Could you check a few things on this model? Use its own coordinates, in mm. A direction names the side the tool comes from. Give positions to 0.01 mm unless a question says otherwise; leave off trailing zeros. Loops run counter-clockwise (first coordinate to the right, second up) from the corner with the lowest first, then second, coordinate; pieces in that order, holes last. Notation, with made-up numbers: M -31.5,61 L 14.5,61 A31 ccw 14.5,86 Z; hole C 50,36 d7. An arc over 180 degrees is marked long. Answer in a Markdown table with one row per item. Add a question column.
```python
from build123d import *

# Parameters (mm, degrees)
F0_W          = 38
F0_H          = 18.5
F0_R          = 1.5
F0_W_2        = 10
F0_R_2        = 1.75
F1_DEPTH      = 5
F2_W          = 25
F2_H          = 18.5
F3_DEPTH      = 5
F5_DEPTH      = 41.501
F5_DEPTH_BACK = 16.501


with BuildPart() as f1:
    # F0 (on Top) → F1 (new body)
    with BuildSketch(Plane.XY):
        Rectangle(F0_W, F0_H)
        with Locations((-16.65, 0)):
            Circle(F0_R, mode=Mode.SUBTRACT)
        with Locations((16.65, 0)):
            Circle(F0_R, mode=Mode.SUBTRACT)
        with Locations((24, 0)):
            Rectangle(F0_W_2, F0_H)
        with Locations((25, 0)):
            Circle(F0_R_2, mode=Mode.SUBTRACT)
        with Locations((-24, 0)):
            Rectangle(F0_W_2, F0_H)
        with Locations((-25, 0)):
            Circle(F0_R_2, mode=Mode.SUBTRACT)
    extrude(amount=F1_DEPTH)

    # F2 (on face) → F3 (join)
    with BuildSketch(Plane.XY.offset(5)):
        Rectangle(F2_W, F2_H)
    extrude(amount=F3_DEPTH)

    # F4 (on face) → F5 (cut, two sides)
    with BuildSketch(Plane(origin=(-12.5, 0, 0), x_dir=(0, -1, 0), z_dir=(-1, 0, 0))) as f5_sk:
        Polygon((-4.625, 5), (0, 10), (-9.25, 10), (-9.25, 5), align=None)
        Polygon((9.25, 10), (0, 10), (4.625, 5), (9.25, 5), align=None)
        Polygon((9.25, 5), (4.625, 5), (9.25, 0), align=None)
        Polygon((-9.25, 0), (-4.625, 5), (-9.25, 5), align=None)
    extrude(amount=-F5_DEPTH, mode=Mode.SUBTRACT)
    extrude(f5_sk.sketch, amount=F5_DEPTH_BACK, mode=Mode.SUBTRACT)


solid = f1.part
```
Item 1: For faces 4 (the face through (-18.15, 0.07, 2.46)), 5 (the face through (-12.5, 0, 7)), which set-ups out of +Z, -Z, +X, -X, +Y, -Y let a thin tool reach every point of the face, with its end or its side?
Item 2: Suppose I cut it at B-B (x = 25). List the corners of the cut face in (y, z) for me (3 decimals).
Item 3: For P1, Ø3, axis at x = 25, y = 0, coming from the -Z side (3 decimals); P2, Ø2.5, axis at y = 1.5, z = 8.5, coming from the +X side; P3, Ø4, axis at y = 0.5, z = 7.5, coming from the -X side; P4, Ø3, axis at x = 22.5, y = -1, coming from the +Z side, each with a flat end and sliding along its axis, tell me the tip position at first contact or that it passes through.
Item 4: Suppose I cut it at A-A (x = -16.65). List the corners of the cut face in (y, z) for me (3 decimals).
Item 5: I need wall thicknesses on L1, parallel to Z at x = -17, y = 4.25; L2, parallel to Y at x = -16, z = 1.75; L3, parallel to Z at x = -9, y = -5.5. Which ranges of each line are inside material? Lowest first, please.
Item 6: If we mould it in two halves opening along X, with no side actions, what happens to faces 1 (the face through (12.5, 0, 7)), 2 (the face through (-26.75, 0.08, 2.46)), 3 (the face through (21, 0, 5))? For each: +X half, -X half, draft (parallel to the pull), parting line (faces both ways), or undercut.
Item 7: Suppose I cut it at D-D (y = -2.75). List the corners of the cut face in (x, z) for me.
Item 8: Suppose I cut it at C-C (z = 2.75). List the corners of the cut face in (x, y) for me.
Values found:
| question | item | result |
|---|---|---|
| 1 | face 4 | +Z, -Z |
| 1 | face 5 | +Z, -X, +Y, -Y |
| 2 | outline | M -9.25,0 L -1.75,0 L -1.75,5 L -4.625,5 Z; M 1.75,0 L 9.25,0 L 4.625,5 L 1.75,5 Z |
| 3 | P1 | through |
| 3 | P2 | x = 12.5 |
| 3 | P3 | x = -12.5 |
| 3 | P4 | z = 5 |
| 4 | outline | M -9.25,0 L -1.5,0 L -1.5,5 L -4.625,5 Z; M 1.5,0 L 9.25,0 L 4.625,5 L 1.5,5 Z |
| 5 | L1 | 0 to 5 |
| 5 | L2 | -7.63 to -1.35, 1.35 to 7.63 |
| 5 | L3 | 0 to 4.05 |
| 6 | face 1 | +X half |
| 6 | face 2 | undercut |
| 6 | face 3 | draft |
| 7 | outline | M -29,0 L 29,0 L 29,5 L 12.5,5 L 12.5,7.03 L -12.5,7.03 L -12.5,5 L -29,5 Z |
| 8 | outline | M -29,-6.71 L 29,-6.71 L 29,6.71 L -29,6.71 Z; hole C -25,0 d3.5; hole C -16.65,0 d3; hole C 16.65,0 d3; hole C 25,0 d3.5 |
